```python
from build123d import *

# Parameters (mm, degrees)
PLATEFRAME_DEPTH          = 150
SKETCH3_R                 = 2.5
HOLESUPPORT_DEPTH         = 13.5
SKETCH4_R                 = 4.15
SKETCH4_R_2               = 2.15
CYLINDRICALSUPPORTS_DEPTH = 12.5
SKETCH5_W                 = 43
SKETCH5_H                 = 43
SKETCH5_W_2               = 89.65
SKETCH5_H_2               = 57.35
SKETCH5_W_3               = 58
SKETCH5_H_3               = 73
ITEMLAYOUT_DEPTH          = 4
HOLECUTOUT_DEPTH          = 7.5
SKETCH7_R                 = 1.5
HOLERASPBERRYPI_DEPTH     = 3.5
SKETCH8_R                 = 1.85
HOLEMOTORDRIVER_DEPTH     = 3.5
SKETCH10_W                = 45
SKETCH10_H                = 45
SKETCH10_W_2              = 43
SKETCH10_H_2              = 43
CUTMOTORDRIVER_DEPTH      = 4
SKETCH11_W                = 93.65
SKETCH11_H                = 61.35
SKETCH11_W_2              = 89.65
SKETCH11_H_2              = 57.35
CUTPASPBERRYPI_DEPTH      = 4
SKETCH12_W                = 191.6
SKETCH12_H                = 13
SKETCH12_H_2              = 14
CUTPLATEEDGES_DEPTH       = 12.5
SKETCH13_W                = 6.5
SKETCH13_H                = 15
CUTSHELLHOLES_DEPTH       = 12.5
SKETCH14_W                = 51
SKETCH14_H                = 51
CUTMOTORDRIVER2_DEPTH     = 4
SKETCH15_R                = 2.5
STANDOFFHOLES_DEPTH       = 13.5
SKETCH16_W                = 2.5
SKETCH16_H                = 28
CUT_EXTRUDE1_DEPTH        = 5


with BuildPart() as part:
    # Sketch2 → PlateFrame (new body)
    with BuildSketch(Plane.XY):
        Polygon((179.1, 12.5), (191.6, 12.5), (191.6, 5), (184.1, 5), (184.1, 0), (7.5, 0), (7.5, 5), (0, 5), (0, 12.5), (12.5, 12.5), (12.5, 7.5), (179.1, 7.5), align=None)
    extrude(amount=PLATEFRAME_DEPTH)

    # Sketch3 → HoleSupport (cut, through all)
    with BuildSketch(Plane(origin=(0, 12.5, 0), x_dir=(1, 0, 0), z_dir=(0, 1, 0))):
        with Locations((8.05, -66.85)):
            Circle(SKETCH3_R)
        with Locations((8.05, -83.15)):
            Circle(SKETCH3_R)
        with Locations((183.55, -66.85)):
            Circle(SKETCH3_R)
        with Locations((183.55, -83.15)):
            Circle(SKETCH3_R)
    extrude(amount=-HOLESUPPORT_DEPTH, mode=Mode.SUBTRACT)

    # Sketch4 → CylindricalSupports (add)
    with BuildSketch(Plane(origin=(0, 12.5, 0), x_dir=(1, 0, 0), z_dir=(0, 1, 0))):
        with Locations((183.55, -66.85)):
            Circle(SKETCH4_R)
        with Locations((183.55, -66.85)):
            Circle(SKETCH4_R_2, mode=Mode.SUBTRACT)
        with Locations((183.55, -83.15)):
            Circle(SKETCH4_R)
        with Locations((183.55, -83.15)):
            Circle(SKETCH4_R_2, mode=Mode.SUBTRACT)
        with Locations((8.05, -66.85)):
            Circle(SKETCH4_R)
        with Locations((8.05, -66.85)):
            Circle(SKETCH4_R_2, mode=Mode.SUBTRACT)
        with Locations((8.05, -83.15)):
            Circle(SKETCH4_R)
        with Locations((8.05, -83.15)):
            Circle(SKETCH4_R_2, mode=Mode.SUBTRACT)
    extrude(amount=-CYLINDRICALSUPPORTS_DEPTH)

    # Sketch5 → ItemLayout (cut)
    with BuildSketch(Plane(origin=(0, 7.5, 0), x_dir=(1, 0, 0), z_dir=(0, 1, 0))):
        with Locations((39, -108.5)):
            Rectangle(SKETCH5_W, SKETCH5_H)
        with Locations((62.325, -48.675)):
            Rectangle(SKETCH5_W_2, SKETCH5_H_2)
        with Locations((145.1, -56.5)):
            Rectangle(SKETCH5_W_3, SKETCH5_H_3)
    extrude(amount=-ITEMLAYOUT_DEPTH, mode=Mode.SUBTRACT)

    # Sketch6 → HoleCutout (cut)
    with BuildSketch(Plane(origin=(0, 7.5, 0), x_dir=(1, 0, 0), z_dir=(0, 1, 0))):
        Polygon((67.1, -84), (110.1, -84), (110.1, -99), (174.1, -99), (174.1, -130), (110.1, -130), (67.1, -130), align=None)
    extrude(amount=-HOLECUTOUT_DEPTH, mode=Mode.SUBTRACT)

    # Sketch7 → HoleRaspberryPi (cut)
    with BuildSketch(Plane(origin=(0, 3.5, 0), x_dir=(1, 0, 0), z_dir=(0, 1, 0))):
        with Locations((23.26, -23.5)):
            Circle(SKETCH7_R)
        with Locations((23.26, -72.5)):
            Circle(SKETCH7_R)
        with Locations((81.26, -72.5)):
            Circle(SKETCH7_R)
        with Locations((81.26, -23.5)):
            Circle(SKETCH7_R)
    extrude(amount=-HOLERASPBERRYPI_DEPTH, mode=Mode.SUBTRACT)

    # Sketch8 → HoleMotorDriver (cut)
    with BuildSketch(Plane(origin=(0, 3.5, 0), x_dir=(1, 0, 0), z_dir=(0, 1, 0))):
        with Locations((57.56, -127.24)):
            Circle(SKETCH8_R)
        with Locations((57.56, -89.86)):
            Circle(SKETCH8_R)
        with Locations((20.81, -89.86)):
            Circle(SKETCH8_R)
        with Locations((20.81, -127.24)):
            Circle(SKETCH8_R)
    extrude(amount=-HOLEMOTORDRIVER_DEPTH, mode=Mode.SUBTRACT)

    # Sketch10 → CutMotorDriver (cut)
    with BuildSketch(Plane(origin=(0, 7.5, 0), x_dir=(1, 0, 0), z_dir=(0, 1, 0))):
        with Locations((39, -108.5)):
            Rectangle(SKETCH10_W, SKETCH10_H)
        with Locations((39, -108.5)):
            Rectangle(SKETCH10_W_2, SKETCH10_H_2, mode=Mode.SUBTRACT)
    extrude(amount=-CUTMOTORDRIVER_DEPTH, mode=Mode.SUBTRACT)

    # Sketch11 → CutPaspberryPi (cut)
    with BuildSketch(Plane(origin=(0, 7.5, 0), x_dir=(1, 0, 0), z_dir=(0, 1, 0))):
        with Locations((62.325, -48.675)):
            Rectangle(SKETCH11_W, SKETCH11_H)
        with Locations((62.325, -48.675)):
            Rectangle(SKETCH11_W_2, SKETCH11_H_2, mode=Mode.SUBTRACT)
    extrude(amount=-CUTPASPBERRYPI_DEPTH, mode=Mode.SUBTRACT)

    # Sketch12 → CutPlateEdges (cut)
    with BuildSketch(Plane(origin=(0, 12.5, 0), x_dir=(1, 0, 0), z_dir=(0, 1, 0))):
        with Locations((95.8, -6.5)):
            Rectangle(SKETCH12_W, SKETCH12_H)
        with Locations((95.8, -143)):
            Rectangle(SKETCH12_W, SKETCH12_H_2)
    extrude(amount=-CUTPLATEEDGES_DEPTH, mode=Mode.SUBTRACT)

    # Sketch13 → CutShellHoles (cut)
    with BuildSketch(Plane(origin=(0, 12.5, 0), x_dir=(1, 0, 0), z_dir=(0, 1, 0))):
        with Locations((6.25, -51.85)):
            Rectangle(SKETCH13_W, SKETCH13_H)
        with Locations((6.25, -98.15)):
            Rectangle(SKETCH13_W, SKETCH13_H)
        with Locations((185.35, -51.85)):
            Rectangle(SKETCH13_W, SKETCH13_H)
        with Locations((185.35, -98.15)):
            Rectangle(SKETCH13_W, SKETCH13_H)
    extrude(amount=-CUTSHELLHOLES_DEPTH, mode=Mode.SUBTRACT)

    # Sketch14 → CutMotorDriver2 (cut)
    with BuildSketch(Plane(origin=(0, 7.5, 0), x_dir=(1, 0, 0), z_dir=(0, 1, 0))):
        with Locations((39, -108.5)):
            Rectangle(SKETCH14_W, SKETCH14_H)
    extrude(amount=-CUTMOTORDRIVER2_DEPTH, mode=Mode.SUBTRACT)

    # Sketch15 → StandoffHoles (cut, through all)
    with BuildSketch(Plane(origin=(0, 12.5, 0), x_dir=(1, 0, 0), z_dir=(0, 1, 0))):
        with Locations((4.5, -36.85)):
            Circle(SKETCH15_R)
        with Locations((4.5, -113.15)):
            Circle(SKETCH15_R)
        with Locations((187.1, -113.15)):
            Circle(SKETCH15_R)
        with Locations((187.1, -36.85)):
            Circle(SKETCH15_R)
    extrude(amount=-STANDOFFHOLES_DEPTH, mode=Mode.SUBTRACT)

    # Sketch16 → Cut-Extrude1 (cut)
    with BuildSketch(Plane.XZ):
        with Locations((8.75, 122)):
            Rectangle(SKETCH16_W, SKETCH16_H)
        with Locations((182.85, 122)):
            Rectangle(SKETCH16_W, SKETCH16_H)
        with Locations((182.85, 27)):
            Rectangle(SKETCH16_W, SKETCH16_H)
        with Locations((8.75, 27)):
            Rectangle(SKETCH16_W, SKETCH16_H)
    extrude(amount=-CUT_EXTRUDE1_DEPTH, mode=Mode.SUBTRACT)


solid = part.part
```
Here's how the part is built. I have some questions about the finished solid (model axes, mm). A direction names the side the tool comes from. Round coordinates to 2 decimals unless told otherwise and drop trailing zeros. Order: outer loops, then holes, each group sorted by start corner. A loop starts at its lowest first (then second) coordinate and runs counter-clockwise, first axis right, second up. Notation, with made-up numbers: M 47.25,-18 L 75.25,-18 A24 ccw 75.25,15 Z; hole C 41.5,-26.75 d10. An arc over 180 degrees is marked long. One line per question, with ' | ' between items.
1) I want a section at B-B, the plane z = 95. Write out the boundary of the cut face in (x, y).
Working result:
outline: M 0,5 L 3,5 L 3,12.5 L 0,12.5 Z; M 9.5,0 L 67.1,0 L 67.1,7.5 L 64.5,7.5 L 64.5,3.5 L 13.5,3.5 L 13.5,7.5 L 12.5,7.5 L 12.5,12.5 L 9.5,12.5 Z; M 110.1,0 L 182.1,0 L 182.1,12.5 L 179.1,12.5 L 179.1,7.5 L 110.1,7.5 Z; M 188.6,5 L 191.6,5 L 191.6,12.5 L 188.6,12.5 Z
2) I want a section at A-A, the plane y = 10. State how many separate pieces and enclosed holes the cut face has, then the cut area to 3 significant figures.
Working result:
separate pieces: 2 | enclosed holes: 12 | area: 2,550 mm²
3) For pin 1 Ø2 at (x, z) = (91, 29) entering from +Y; pin 2 Ø12 at (x, z) = (117, 71) entering from +Y; pin 3 Ø2.5 at (y, z) = (3.5, 107.5) entering from +X, each with a flat end and sliding along its axis, tell me the tip position at first contact or that it passes through.
Working result:
pin 1: y = 3.5 | pin 2: y = 7.5 | pin 3: x = 184.1
4) For faces 1 (the face through (39, 6, 83)), 2 (the face through (174.1, 4, 114)), 3 (the face through (114, 7.5, 61)), which set-ups out of +Z, -Z, +X, -X, +Y, -Y let a thin tool reach every point of the face, with its end or its side?
Working result:
face 1: +Y | face 2: +Y, -Y | face 3: +Z, -Z, +Y
5) I need wall thicknesses on line 1 along X through (y, z) = (2.3, 89.86); line 2 along X through (y, z) = (8.25, 52.5); line 3 along Z through (x, y) = (147, 5.25). Which ranges of each line are inside material? Lowest first, please.
Working result:
line 1: 7.5 to 18.96, 22.66 to 55.71, 59.41 to 67.1, 110.1 to 184.1 | line 2: 0 to 3, 9.5 to 12.5, 179.1 to 182.1, 188.6 to 191.6 | line 3: 13 to 20, 93 to 99, 130 to 136
6) I want a section at C-C, the plane x = 105.5. Write out the boundary of the cut face in (y, z).
Working result:
outline: M 0,13 L 7.5,13 L 7.5,18 L 3.5,18 L 3.5,79.35 L 7.5,79.35 L 7.5,84 L 0,84 Z; M 0,130 L 7.5,130 L 7.5,136 L 0,136 Z
7) If we mould it in two halves opening along Z, with no side actions, what happens to faces 4 (the face through (181.6, 2, 122)), 5 (the face through (5.84, 8.8, 34.74)), 6 (the face through (94, 5, 136))? For each: +Z half, -Z half, draft (parallel to the pull), parting line (faces both ways), or undercut.
Working result:
face 4: draft | face 5: undercut | face 6: +Z half
8) I want a section at D-D, the plane z = 66.85. Write out the boundary of the cut face in (x, y), then the cut area to 3 significant figures.
Working result:
outline: M 0,5 L 3.9,5 L 3.9,0 L 5.9,0 L 5.9,12.5 L 0,12.5 Z; M 10.2,0 L 181.4,0 L 181.4,12.5 L 179.1,12.5 L 179.1,7.5 L 174.1,7.5 L 174.1,3.5 L 116.1,3.5 L 116.1,7.5 L 109.15,7.5 L 109.15,3.5 L 15.5,3.5 L 15.5,7.5 L 12.5,7.5 L 12.5,12.5 L 10.2,12.5 Z; M 185.7,0 L 187.7,0 L 187.7,5 L 191.6,5 L 191.6,12.5 L 185.7,12.5 Z | area: 809 mm²
